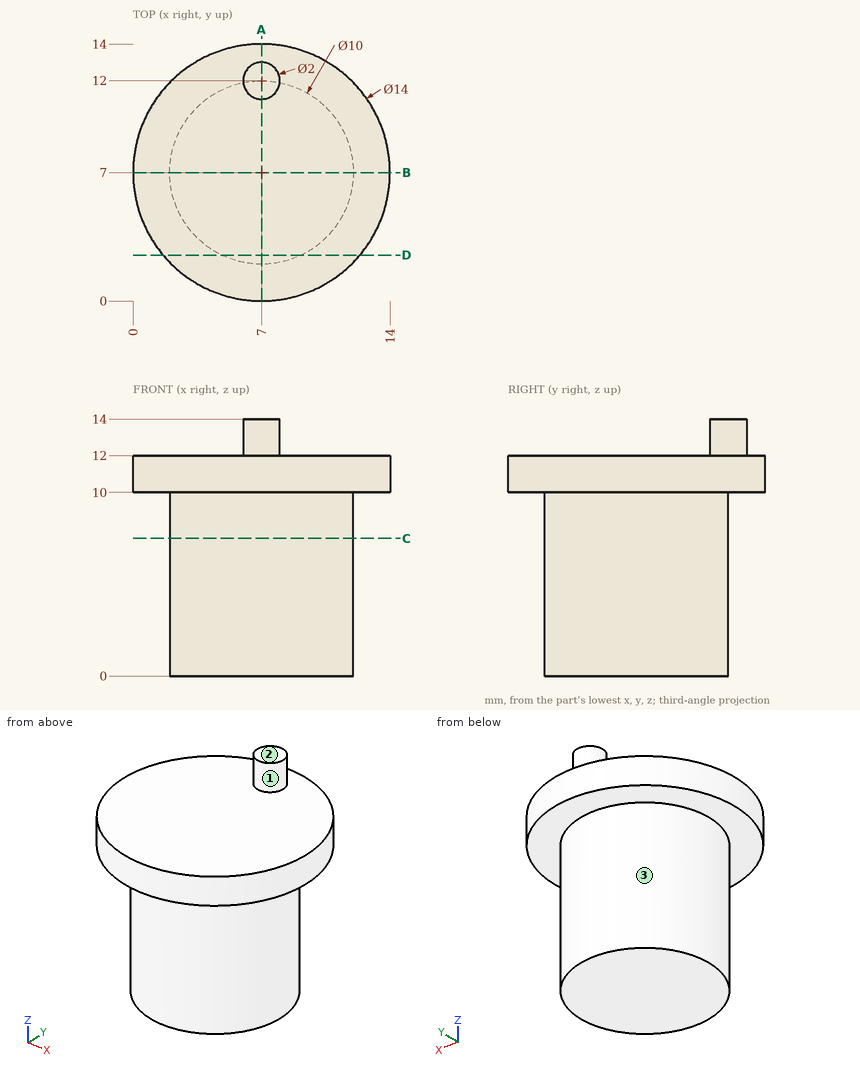
Input: dimensioned drawing with shaded views. Units: mm. Origin: part minimum x, y, z. A direction names the side the tool comes from. Round coordinates to 2 decimals unless told otherwise and drop trailing zeros. Order: outer loops, then holes, each group sorted by start corner. A loop starts at its lowest first (then second) coordinate and runs counter-clockwise, first axis right, second up. Notation, with made-up numbers: (-8.5, 86) -> (18.5, 86) arc R30 cw to (18.5, 113) -> close; hole circle Ø10 at (33, 78.5). An arc over 180 degrees is marked (long way). One line per item, written item: value. Start each with the question number.
Q1. Section query B-B (y = 7). Return the cut outline in (x, z), plus the area to 3 significant figures.
Q2. Pin query (flat end, axial travel): pin 1 (8 mm diameter, centred on x = 9, y = 2, fed in from +Z); pin 2 (2 mm diameter, centred on x = 12.5, y = 10, fed in from -Z); pin 3 (3 mm diameter, centred on x = 4.5, z = 10.5, fed in from +Y). Return the tip coordinate at first contact, or that it passes through.
Q3. Section query C-C (z = 7.5). Return the cut outline in (x, y), plus the area to 3 significant figures.
Q4. Access query for the marked faces 1, 2 and 3. Directions: +Z, -Z, +X, -X, +Y, -Y. A direction counts if a zero-diameter tool reaches every point of the face in a straight line with its end or side. Return the directions, or none.
Q5. Material intervals for probe 1 along Z at (x, y) = (11.25, 10.25); probe 2 along Z at (x, y) = (6.5, 4.25); probe 3 along Y at (x, z) = (2.25, 11.5), sorted ascending.
Q6. Section query A-A (x = 7). Return the cut outline in (y, z).
Q7. Section query D-D (y = 2.5). Return the cut outline in (x, z), plus the area to 3 significant figures.
Findings below:
1. outline: (0, 10) -> (2, 10) -> (2, 0) -> (12, 0) -> (12, 10) -> (14, 10) -> (14, 12) -> (0, 12) -> close
1. area: 128 mm²
2. pin 1: z = 12
2. pin 2: z = 10
2. pin 3: y = 13.93
3. outline: circle Ø10 at (7, 7)
3. area: 78.5 mm²
4. face 1: +Z
4. face 2: +Z, +X, -X, +Y, -Y
4. face 3: -Z
5. probe 1: 10 to 12
5. probe 2: 0 to 12
5. probe 3: 1.86 to 12.14
6. outline: (0, 10) -> (2, 10) -> (2, 0) -> (12, 0) -> (12, 10) -> (14, 10) -> (14, 12) -> (13, 12) -> (13, 14) -> (11, 14) -> (11, 12) -> (0, 12) -> close
7. outline: (1.64, 10) -> (4.82, 10) -> (4.82, 0) -> (9.18, 0) -> (9.18, 10) -> (12.36, 10) -> (12.36, 12) -> (1.64, 12) -> close
7. area: 65.0 mm²
